The model under review builds one solid part; all positions refer to its coordinate system, in mm. Round coordinates to 2 decimals unless told otherwise and drop trailing zeros. Loops run counter-clockwise (first coordinate to the right, second up) from the corner with the lowest first, then second, coordinate; pieces in that order, holes last. Notation, with made-up numbers: M -7,61 L 28,61 A14 ccw 28,76 Z; hole C 31,-38.75 d7. An arc over 180 degrees is marked long. Answer as a JSON object with one key per item and string values. Group by question number.
Item 1: To check wall thickness, follow line 1 (Y direction, x = 194, z = -17.75); line 2 (X direction, y = -0.5, z = -19.05). State the ranges of each line that lie inside material, in increasing order.
Item 2: Consider section C-C (z = -11). Give the boundary of the cut face in (x, y).
Item 3: Insertion check: P1, Ø10, axis at x = 111, y = -8.5, coming from the +Z side. The pin has a flat end and moves straight along its axis. Give the tip position at first contact, or say it passes through.
Item 4: Consider section A-A (x = 596.9). Give the boundary of the cut face in (y, z).
Item 5: Consider section B-B (x = 458). Give the boundary of the cut face in (y, z).
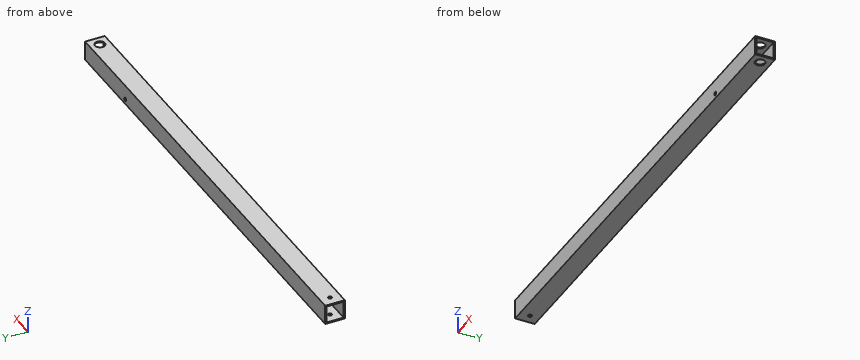
```python
from build123d import *

# Parameters (mm, degrees)
SKETCH1_W                = 609.6
SKETCH1_H                = 25.4
BOSS_EXTRUDE1_DEPTH      = 25.4
SKETCH2_W                = 22.225
SKETCH2_H                = 22.225
CUT_EXTRUDE1_DEPTH       = 611.657416233
HOLE1_D                  = 4.8006
HOLE1_DEPTH              = 1.5875
M4_CLEARANCE_HOLE1_D     = 4.7625
M4_CLEARANCE_HOLE1_DEPTH = 1.5875
HOLE2_D                  = 12.7
HOLE2_DEPTH              = 1.5875
M4_CLEARANCE_HOLE2_D     = 4.7625
M4_CLEARANCE_HOLE2_DEPTH = 25.4
HOLE3_D                  = 12.7
HOLE3_DEPTH              = 25.4
HOLE4_D                  = 4.8006
HOLE4_DEPTH              = 25.4


with BuildPart() as part:
    # Sketch1 → Boss-Extrude1 (new body)
    with BuildSketch(Plane.XY):
        with Locations((304.8, -12.7)):
            Rectangle(SKETCH1_W, SKETCH1_H)
    extrude(amount=-BOSS_EXTRUDE1_DEPTH)

    # Sketch2 → Cut-Extrude1 (cut, through all)
    with BuildSketch(Plane.ZY):
        with Locations((-12.7, -12.7)):
            Rectangle(SKETCH2_W, SKETCH2_H)
    extrude(amount=-CUT_EXTRUDE1_DEPTH, mode=Mode.SUBTRACT)

    # Hole1
    with Locations(Plane(origin=(0, -23.8125, 0), x_dir=(1, 0, 0), z_dir=(0, 1, 0))):
        with Locations((508, 19.05)):
            Hole(HOLE1_D / 2, depth=HOLE1_DEPTH)

    # M4 Clearance Hole1
    with Locations(Plane.XY.offset(-23.8125)):
        with Locations((12.7, -12.7)):
            Hole(M4_CLEARANCE_HOLE1_D / 2, depth=M4_CLEARANCE_HOLE1_DEPTH)

    # Hole2
    with Locations(Plane.XY.offset(-23.8125)):
        with Locations((596.9, -12.7)):
            Hole(HOLE2_D / 2, depth=HOLE2_DEPTH)

    # M4 Clearance Hole2
    with Locations(Plane.XY):
        with Locations((12.7, -12.7)):
            Hole(M4_CLEARANCE_HOLE2_D / 2, depth=M4_CLEARANCE_HOLE2_DEPTH)

    # Hole3
    with Locations(Plane.XY):
        with Locations((596.9, -12.7)):
            Hole(HOLE3_D / 2, depth=HOLE3_DEPTH)

    # Hole4
    with Locations(Plane(origin=(0, 0, 0), x_dir=(1, 0, 0), z_dir=(0, 1, 0))):
        with Locations((508, 19.05)):
            Hole(HOLE4_D / 2, depth=HOLE4_DEPTH)


solid = part.part
```
Geometry results:
{
 "1": {"line 1": "y = -25.4 to -23.81, -1.59 to 0", "line 2": "x = 0 to 505.6, 510.4 to 609.6"},
 "2": {"outline": "M 0,-25.4 L 609.6,-25.4 L 609.6,-23.81 L 0,-23.81 Z; M 0,-1.59 L 609.6,-1.59 L 609.6,0 L 0,0 Z"},
 "3": {"P1": "stops at z = 0"},
 "4": {"outline": "M -25.4,-25.4 L -19.05,-25.4 L -19.05,-23.81 L -23.81,-23.81 L -23.81,-1.59 L -19.05,-1.59 L -19.05,0 L -25.4,0 Z; M -6.35,-25.4 L 0,-25.4 L 0,0 L -6.35,0 L -6.35,-1.59 L -1.59,-1.59 L -1.59,-23.81 L -6.35,-23.81 Z"},
 "5": {"outline": "M -25.4,-25.4 L 0,-25.4 L 0,0 L -25.4,0 Z; hole M -23.81,-23.81 L -1.59,-23.81 L -1.59,-1.59 L -23.81,-1.59 Z"}
}
